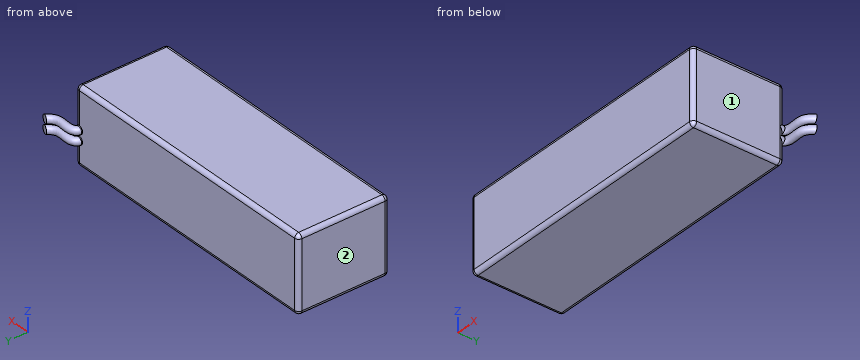
```python
from build123d import *

# Parameters (mm, degrees)
SZKIC1_W                         = 138
SZKIC1_H                         = 38
DODANIE_WYCI_GNI_CIE1_DEPTH      = 46
ZAOKR_GLENIE1_R                  = 2
DODANIE_WYCI_GNI_CIE2_REACH      = 87.348
DODANIE_WYCI_GNI_CIE2_END_RADIUS = 2
SZKIC3_R                         = 2
SZKIC5_R                         = 2


with BuildPart() as part:
    # Szkic1 → Dodanie-wyciągnięcie1 (new body)
    with BuildSketch(Plane(origin=(0, 0, 0), x_dir=(1, 0, 0), z_dir=(0, 1, 0))):
        Rectangle(SZKIC1_W, SZKIC1_H)
    extrude(amount=DODANIE_WYCI_GNI_CIE1_DEPTH)

    # Zaokrąglenie1
    zaokr_glenie1_edges = [part.edges().sort_by_distance(p)[0] for p in [
        (-69, 46, 0),
        (0, 46, 19),
        (69, 46, 0),
        (0, 0, 19),
        (-69, 0, 0),
        (0, 0, -19),
        (69, 0, 0),
        (69, 23, 19),
        (-69, 23, 19),
        (-69, 23, -19),
        (69, 23, -19),
        (0, 46, -19),
    ]]
    fillet(zaokr_glenie1_edges, radius=ZAOKR_GLENIE1_R)

    # Dodanie-wyciągnięcie2: up to this cylinder (the profile starts outside it)
    dodanie_wyci_gni_cie2_end = Plane(origin=(67, 44, -4), z_dir=(0, 0, -1)) * Cylinder(DODANIE_WYCI_GNI_CIE2_END_RADIUS, 184.696, mode=Mode.PRIVATE)
    # Szkic3 → Dodanie-wyciągnięcie2 (add, up to the surface)
    with BuildSketch(Plane(origin=(0, 46.5, 0), x_dir=(1, 0, 0), z_dir=(0, 1, 0)), mode=Mode.PRIVATE) as dodanie_wyci_gni_cie2_sk1:
        with Locations(Location((67, 6.5, 0), (0, 0, 270))):
            Circle(SZKIC3_R)
    dodanie_wyci_gni_cie2_tool1 = extrude(dodanie_wyci_gni_cie2_sk1.sketch, amount=-DODANIE_WYCI_GNI_CIE2_REACH, mode=Mode.PRIVATE) - dodanie_wyci_gni_cie2_end
    add(dodanie_wyci_gni_cie2_tool1.solids().sort_by_distance((67, 46.5, -6.5))[0])
    # Szkic3 → Dodanie-wyciągnięcie2 (add, up to the surface)
    with BuildSketch(Plane(origin=(0, 46.5, 0), x_dir=(1, 0, 0), z_dir=(0, 1, 0)), mode=Mode.PRIVATE) as dodanie_wyci_gni_cie2_sk2:
        with Locations(Location((67, 1.5, 0), (0, 0, 270))):
            Circle(SZKIC3_R)
    dodanie_wyci_gni_cie2_tool2 = extrude(dodanie_wyci_gni_cie2_sk2.sketch, amount=-DODANIE_WYCI_GNI_CIE2_REACH, mode=Mode.PRIVATE) - dodanie_wyci_gni_cie2_end
    add(dodanie_wyci_gni_cie2_tool2.solids().sort_by_distance((67, 46.5, -1.5))[0])

    # Wyciągnięcie po ścieżce1: sweep along a path in Szkic4
    with BuildLine() as wyci_gni_cie_po_cie_ce1_path:  # in the path sketch's own coordinates; laid on its plane below (add() does not lay a ready-made edge on the line's plane)
        add(Edge.make_bspline(
            [(-67, 46.5), (-67.812300982, 48.700029071), (-76.558056505, 48.053598024), (-78.81196866, 48.196334496), (-81.546543778, 51.620091174)],
            knots=[0, 0, 0, 0, 0.368299585, 1, 1, 1, 1], degree=3))
    # Szkic5 → Wyciągnięcie po ścieżce1 (sweep)
    with BuildSketch(Plane(origin=(0, 46.5, 0), x_dir=(1, 0, 0), z_dir=(0, 1, 0))):
        with Locations((67, 6.5)):
            Circle(SZKIC5_R)
        with Locations((67, 1.5)):
            Circle(SZKIC5_R)
    sweep(path=Plane(origin=(0, 0, -4), x_dir=(-1, 0, 0), z_dir=(0, 0, -1)) * wyci_gni_cie_po_cie_ce1_path.line)


solid = part.part
```
Model file for the job. Use its own axes, mm. Face numbers are marked on the shaded views. A direction names the side the tool comes from. Coordinates: 2 decimals unless noted, no trailing zeros. Write each loop counter-clockwise with the first axis right and the second up, starting at its lowest first coordinate (ties: lowest second). Pieces come first, ordered by that corner, then holes. Notation, with made-up numbers: (-27, 57) - (-7, 57) arc R8 ccw to (-7, 71) - close; hole circle Ø5 at (72, -28). An arc over 180 degrees is marked (long way). One line per item, written item: value. Start each with the question number.
1. Slice it at B-B (z = 7.5). Write the cut outline in (x, y).
2. Probe line 1 (Z direction, x = 72, y = 48.5); line 2 (X direction, y = 11, z = 4.5); line 3 (Y direction, x = -35.5, z = -13). List the from-to ranges inside material, lowest first. Write a range as from..to.
3. Slice it at A-A (x = -53). Write the cut outline in (y, z), plus the area to 3 significant figures.
4. Tool access for the marked faces 1 and 2: list every direction of +Z, -Z, +X, -X, +Y, -Y with a clear straight run to the whole face (end or side of a thin tool).
5. Flat gauge pins, fed straight in: pin 1 (2 mm diameter, centred on y = 38, z = 1, fed in from +X); pin 2 (1 mm diameter, centred on x = -22.5, y = 44.5, fed in from -Z); pin 3 (3 mm diameter, centred on x = -40.5, y = 46.5, fed in from -Z). Where does each tip first touch, or does it go through?
Answers below:
1. outline: (-69, 2) arc R2 ccw to (-67, 0) - (67, 0) arc R2 ccw to (69, 2) - (69, 44) arc R2 ccw to (67, 46) - (-67, 46) arc R2 ccw to (-69, 44) - close
2. line 1: z = -8.5..-4.5, -3.5..0.5
2. line 2: x = -69..69
2. line 3: y = 0..46
3. outline: (0, -17) arc R2 ccw to (2, -19) - (44, -19) arc R2 ccw to (46, -17) - (46, 17) arc R2 ccw to (44, 19) - (2, 19) arc R2 ccw to (0, 17) - close
3. area: 1,740 mm^2
4. face 1: +Z, -Z, +X, -Y
4. face 2: +Z, -Z, -X, +Y, -Y
5. pin 1: stops at x = 69
5. pin 2: stops at z = -19
5. pin 3: stops at z = -18.73
